Autodesk Inventor part; units mm, degrees
ref_plane "YZ Plane" through (0, 0, 0) normal (1, 0, 0) x (0, 1, 0)
ref_plane "XZ Plane" through (0, 0, 0) normal (0, 1, 0) x (-1, 0, 0)
ref_plane "XY Plane" through (0, 0, 0) normal (0, 0, 1) x (1, 0, 0)
sketch "Sketch1" plane through (0, 0, 0) normal (0, 0, 1) x (1, 0, 0)
  line L0 (-65.00021, 64.999866) -> (65.00021, 64.999866)
  line L1 (65.00021, 64.999866) -> (65.00021, -64.999866)
  line L2 (65.00021, -64.999866) -> (-65.00021, -64.999866)
  line L3 (-65.00021, -64.999866) -> (-65.00021, 64.999866)
  line L4 (-65.00021, 64.999866) -> (65.00021, -64.999866) construction
  line L5 (65.00021, 64.999866) -> (-65.00021, -64.999866) construction
  line L6 (29.999974, -64.999866) -> (65.00021, -29.999445)
  line L7 (-29.999622, -64.999866) -> (-65.00021, -29.999464)
  line L8 (-29.999622, 64.999866) -> (-65.00021, 29.999464)
  line L9 (29.998617, 64.999866) -> (65.00021, 29.998087)
  line L10 (-13.50021, 64.999866) -> (116.50021, -64.999866) construction
  line L11 (64.999934, -10.4998) -> (38.000066, -10.4998)
  line L12 (38.000066, -10.4998) -> (38.000066, 10.4998)
  line L13 (38.000066, 10.4998) -> (64.999934, 10.4998)
  line L14 (64.999934, 10.4998) -> (64.999934, -10.4998)
  line L15 (64.999934, -10.4998) -> (38.000066, 10.4998) construction
  line L16 (38.000066, -10.4998) -> (64.999934, 10.4998) construction
  line L17 (-38.000066, -10.4998) -> (-64.999934, -10.4998)
  line L18 (-64.999934, -10.4998) -> (-64.999934, 10.4998)
  line L19 (-64.999934, 10.4998) -> (-38.000066, 10.4998)
  line L20 (-38.000066, 10.4998) -> (-38.000066, -10.4998)
  line L21 (-38.000066, -10.4998) -> (-64.999934, 10.4998) construction
  line L22 (-64.999934, -10.4998) -> (-38.000066, 10.4998) construction
  line L23 (16.970375, 2.121415) -> (-2.121415, -16.970375)
  line L24 (-2.121415, -16.970375) -> (-16.970375, -2.121415)
  line L25 (-16.970375, -2.121415) -> (2.121415, 16.970375)
  line L26 (2.121415, 16.970375) -> (16.970375, 2.121415)
  line L27 (-2.121415, -16.970375) -> (2.121415, 16.970375) construction
extrude "Extrusion1" add sketch "Sketch1" along normal blind 2 contours L0 L9 L1 L13 L12 L11 L6 L2 L7 L3 L17 L20 L19 L8 | L19 L20 L17 L3 | L1 L11 L12 L13 | L23 L24 L25 L26
sketch "Sketch2" plane through (0, 0, 2) normal (0, 0, 1) x (1, 0, 0)
  circle A0 centre (22, 60) radius 1.499868
  circle A1 centre (-22, 60) radius 1.499868
  circle A2 centre (22, -60) radius 1.499868
  circle A3 centre (-22, -60) radius 1.499868
  circle A4 centre (55, 18) radius 1.499868
  circle A5 centre (55, -18) radius 1.499868
  circle A6 centre (-55, 18) radius 1.499868
  circle A7 centre (-54.942641, 18) radius 1.499868
  circle A8 centre (-55, -18) radius 1.499868
  circle A9 centre (-54.942641, -18) radius 1.499868
  point P0 (-54.971321, 16.500406)
  point P1 (-54.971321, 19.499594)
  point P2 (-54.971321, -19.499594)
  point P3 (-54.971321, -16.500406)
extrude "Extrusion2" cut sketch "Sketch2" against normal blind 10
sketch "Sketch1 outline for Extrusion3" plane through (0, 0, 0) normal (0, 0, 1) x (1, 0, 0)
  line L0 (64.999934, -10.4998) -> (64.999934, 10.4998)
  line L1 (38.000066, -10.4998) -> (64.999934, -10.4998)
  line L2 (38.000066, 10.4998) -> (38.000066, -10.4998)
  line L3 (64.999934, 10.4998) -> (38.000066, 10.4998)
extrude "Extrusion3" cut sketch "Sketch1 outline for Extrusion3" along normal blind 10
properties part number "t960_power_distribution_board_TL2996_bottom"
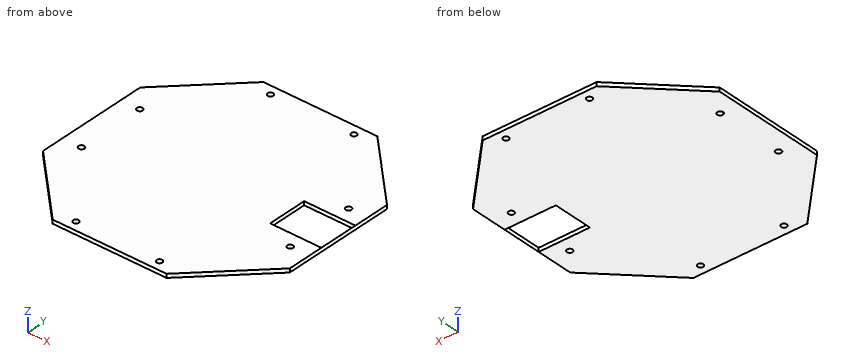
Can you work these out from the model? Positions are in its coordinate system, mm. Give positions to 0.01 mm unless a question says otherwise; leave off trailing zeros. Order: outer loops, then holes, each group sorted by start corner. A loop starts at its lowest first (then second) coordinate and runs counter-clockwise, first axis right, second up. Notation, with made-up numbers: M 31,-1 L 63,-1 A17 cw 63,10 Z; hole C -19.75,36 d2. An arc over 180 degrees is marked long. Use one line per item in the form item = value.
Item 1: If I drill on line 1 along Y through (x, z) = (-22, 0.6); line 2 along Y through (x, z) = (55, 1.45); line 3 along X through (y, z) = (-18.5, 0.3), over which ranges is the centre line in solid material (lowest first)? Write a range as [from, to].
Values follow:
line_1 = [-65, -61.5], [-58.5, 58.5], [61.5, 65]
line_2 = [-40, -19.5], [-16.5, -10.5], [10.5, 16.5], [19.5, 40]
line_3 = [-65, -56.41], [-53.53, 53.59], [56.41, 65]
Item 2: If we section it at C-C, the plane x = 55: Write out the boundary of the cut face in (y, z), and give its area (3 significant figures).
Values follow:
outline = M -40,0 L -19.5,0 L -19.5,2 L -40,2 Z; M -16.5,0 L -10.5,0 L -10.5,2 L -16.5,2 Z; M 10.5,0 L 16.5,0 L 16.5,2 L 10.5,2 Z; M 19.5,0 L 40,0 L 40,2 L 19.5,2 Z
area = 106 mm^2
Item 3: If we section it at D-D, the plane z = 1.7: Count the separate pieces of the cut face and the enclosed holes in it, and give its area (3 significant figures).
Values follow:
separate_pieces = 1
enclosed_holes = 9
area = 13,800 mm^2
Item 4: If we section it at B-B, the plane x = 22: Write out the boundary of the cut face in (y, z).
Values follow:
outline = M -65,0 L -61.5,0 L -61.5,2 L -65,2 Z; M -58.5,0 L 58.5,0 L 58.5,2 L -58.5,2 Z; M 61.5,0 L 65,0 L 65,2 L 61.5,2 Z
Item 5: Will these pins go through, and if not, where does the flat tip stop? pin 1 Ø1.8 at (x, y) = (22, -60) entering from -Z; pin 2 Ø0.6 at (x, z) = (55, 1.5) entering from +Y; pin 3 Ø1 at (x, z) = (51, 1) entering from -Y.
Values follow:
pin_1 = through
pin_2 = 40.3
pin_3 = -44.5
Item 6: If we section it at A-A, the plane y = 18: Write out the boundary of the cut face in (x, z), and give its area (3 significant figures).
Values follow:
outline = M -65,0 L -56.5,0 L -56.5,2 L -65,2 Z; M -53.44,0 L 53.5,0 L 53.5,2 L -53.44,2 Z; M 56.5,0 L 65,0 L 65,2 L 56.5,2 Z
area = 248 mm^2
